Input: part model. Units: mm. Frame: model coordinates. A direction names the side the tool comes from. Give positions to 0.01 mm unless a question says otherwise; leave off trailing zeros. Loops run counter-clockwise (first coordinate to the right, second up) from the corner with the lowest first, then second, coordinate; pieces in that order, holes last. Notation, with made-up numbers: M 41,45.5 L 55,45.5 A19 ccw 55,74.5 Z; hole C 32.25,69 d3. An arc over 180 degrees is marked long. Answer as a JSON object with one key per item and string values. Group by question number.
1) Draft query along Y for faces 1 (the cylindrical face through (-6, 0, 3)), 2 (the flat face through (-11, 22, 6.35)), 3 (the flat face through (0, 63.85, 3)). Return one class per face: +Y half, -Y half, draft (parallel to the pull), parting line (faces both ways), or undercut.
2) First-contact query: P1, Ø3, axis at y = 46.5, z = 3.5, coming from the +X side. Flat tip, straight axial feed; report the tip coordinate or a pass-through.
3) Section query B-B on y = 25. Return loops of the section in (x, z), plus the area to 3 significant figures.
4) Section query D-D on z = 4.5. Count the separate pieces of the cut face and the enclosed holes in it, plus the area to 3 significant figures.
5) Section query A-A on x = 26.15. Return loops of the section in (y, z).
6) Access query for faces 4 (the cylindrical face through (-23.23, 12.31, 3.13)), 5 (the flat face through (21.15, 41, 3)). Directions: +Z, -Z, +X, -X, +Y, -Y. A direction counts if a zero-diameter tool reaches every point of the face in a straight line with its end or side. Return the directions, or none.
7) Ray query, L1, parallel to Y at x = -21.15, z = 2; L2, parallel to Y at x = 0, z = 2.5; L3, parallel to Y at x = 26.15, z = 3.5. Return the intervals inside material, ascending.
8) Section query C-C on x = 0. Return loops of the section in (y, z), plus the area to 3 significant figures.
from build123d import *

# Parameters (mm, degrees)
SKETCH2_W            = 42.3
SKETCH2_H            = 85
SKETCH2_R            = 6
SKETCH2_R_2          = 4
BOSS_EXTRUDE1_DEPTH  = 6.35
BOSS_EXTRUDE2_DEPTH  = 6.35
M4_CLEARANCE_HOLE1_D = 4.5
BOSS_EXTRUDE3_DEPTH  = 6.35
M3_CLEARANCE_HOLE2_D = 3.4


with BuildPart() as part:
    # Sketch2 → Boss-Extrude1 (new body)
    with BuildSketch(Plane.XY):
        with Locations((0, 21.35)):
            Rectangle(SKETCH2_W, SKETCH2_H)
        Circle(SKETCH2_R, mode=Mode.SUBTRACT)
        with Locations((0, 25)):
            Circle(SKETCH2_R_2, mode=Mode.SUBTRACT)
        with Locations((0, 50)):
            Circle(SKETCH2_R_2, mode=Mode.SUBTRACT)
    extrude(amount=BOSS_EXTRUDE1_DEPTH)

    # Sketch8 → Boss-Extrude2 (add)
    with BuildSketch(Plane.XY.offset(6.35)):
        Polygon((-21.15, -21.15), (-51.15, -3.829491924), (-51.15, 46.170508076), (-21.15, 63.85), align=None)
    extrude(amount=-BOSS_EXTRUDE2_DEPTH)

    # M4 Clearance Hole1 (through all)
    with Locations(Plane.XY.offset(6.35)):
        with Locations((-21.15, 13.170508076), (-21.15, 29.170508076), (-45.15, 13.170508076), (-45.15, 29.170508076)):
            Hole(M4_CLEARANCE_HOLE1_D / 2)

    # Sketch11 → Boss-Extrude3 (add)
    with BuildSketch(Plane.XY.offset(6.35)):
        Polygon((21.15, -21.15), (31.15, -21.15), (31.15, 8.85), (21.15, 18.85), align=None)
    extrude(amount=-BOSS_EXTRUDE3_DEPTH)

    # M3 Clearance Hole2 (through all)
    with Locations(Plane.XY.offset(6.35)):
        with Locations((12.15, -16.15), (26.15, -16.15)):
            Hole(M3_CLEARANCE_HOLE2_D / 2)


solid = part.part
Output:
{
 "1": {"face 1": "undercut", "face 2": "draft", "face 3": "+Y half"},
 "2": {"P1": "stops at x = 21.15"},
 "3": {"outline": "M -51.15,0 L -4,0 L -4,6.35 L -51.15,6.35 Z; M 4,0 L 21.15,0 L 21.15,6.35 L 4,6.35 Z", "area": "408 mm^2"},
 "4": {"separate pieces": "1", "enclosed holes": "9", "area": "5,680 mm^2"},
 "5": {"outline": "M -21.15,0 L -17.85,0 L -17.85,6.35 L -21.15,6.35 Z; M -14.45,0 L 13.85,0 L 13.85,6.35 L -14.45,6.35 Z"},
 "6": {"face 4": "+Z, -Z", "face 5": "+Z, -Z, +X, +Y"},
 "7": {"L1": "y = -21.15 to 10.92, 15.42 to 26.92, 31.42 to 63.85", "L2": "y = -21.15 to -6, 6 to 21, 29 to 46, 54 to 63.85", "L3": "y = -21.15 to -17.85, -14.45 to 13.85"},
 "8": {"outline": "M -21.15,0 L -6,0 L -6,6.35 L -21.15,6.35 Z; M 6,0 L 21,0 L 21,6.35 L 6,6.35 Z; M 29,0 L 46,0 L 46,6.35 L 29,6.35 Z; M 54,0 L 63.85,0 L 63.85,6.35 L 54,6.35 Z", "area": "362 mm^2"}
}
